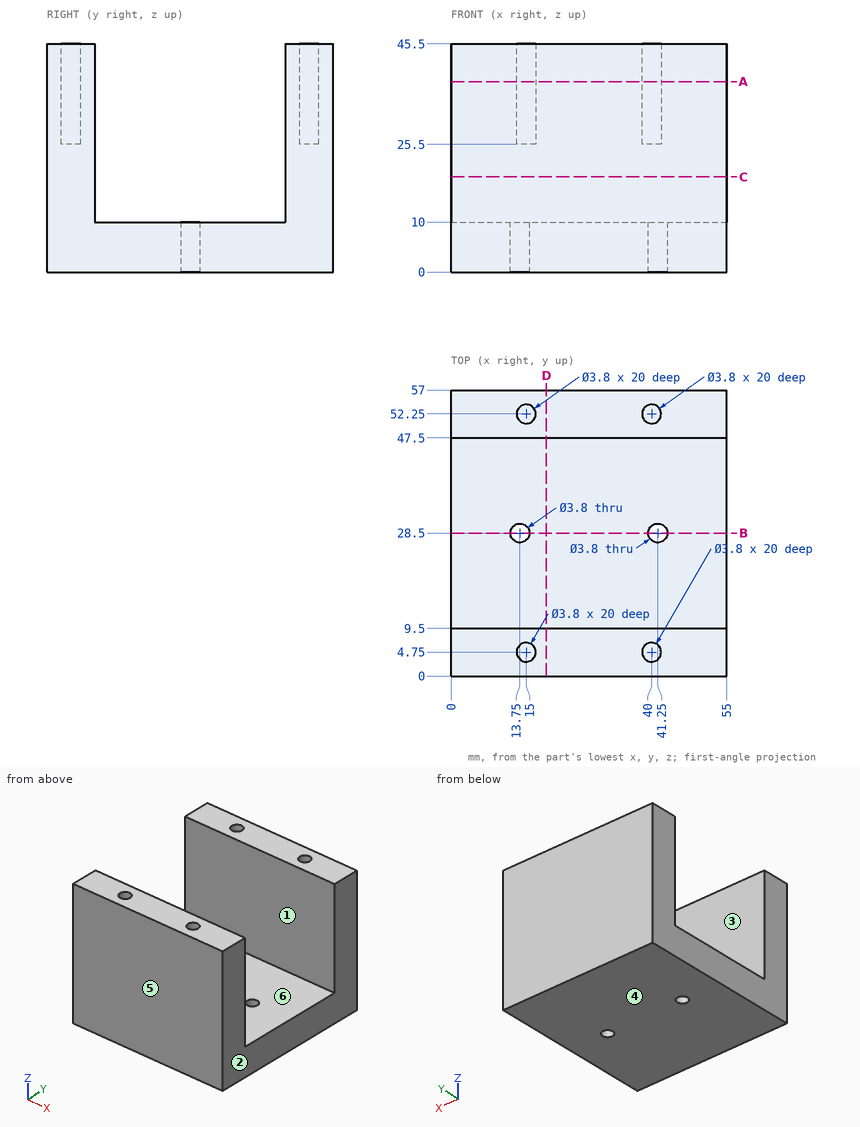
Could you check a few things on this drawing? It's one solid part, dimensions in mm from its lowest x, y, z. A direction names the side the tool comes from. Give positions to 0.01 mm unless a question says otherwise; leave off trailing zeros. Order: outer loops, then holes, each group sorted by start corner. A loop starts at its lowest first (then second) coordinate and runs counter-clockwise, first axis right, second up. Notation, with made-up numbers: (53, -21) - (81, -21) arc R25 ccw to (81, -2) - close; hole circle Ø8 at (47.25, -0.5). An arc over 180 degrees is marked (long way). Return JSON: item names as keys, results as strings. Group by question number.
Q1. Suppose I cut it at A-A, the plane z = 38. Please give me the cut outline in (x, y), and give its area (4 significant figures).
Q2. Please list where these lines run through material, in increasing order: line 1 along Y through (x, z) = (15, 33.75); line 2 along X through (y, z) = (52, 32.5); line 3 along Y through (x, z) = (20, 34). Write a range as [from, to].
Q3. Suppose I cut it at B-B, the plane y = 28.5. Please give me the cut outline in (x, z), and give its area (3 significant figures).
Q4. Thinking about a two-plate mould opening in Y: for the marked faces 3, 4, 5 and 6, which applies, pulls with the +Y half, pulls with the -Y half, needs draft (parallel to the pull), parting line crosses it, or undercut?
Q5. Which directions (+Z, -Z, +X, -X, +Y, -Y) give clear straight access to the entire face, cutting with the end or side of a thin tool? Please do the marked faces 1 and 2.
Q6. Suppose I cut it at C-C, the plane z = 19. Please give me the cut outline in (x, y), and give its area (4 significant figures).
Q7. Will these pins go through, and if not, where does the flat tip stop? pin 1 Ø1 at (x, y) = (41.5, 41.5) entering from +Z; pin 2 Ø6 at (x, y) = (28.5, 12) entering from +Z; pin 3 Ø3.5 at (x, y) = (15, 4.75) entering from +Z; pin 4 Ø3 at (y, z) = (34.5, 13) entering from +X.
Q8. Suppose I cut it at D-D, the plane x = 19. Please give me the cut outline in (y, z).
Resolved:
{
 "1": {"outline": "(0, 0) - (55, 0) - (55, 9.5) - (0, 9.5) - close; (0, 47.5) - (55, 47.5) - (55, 57) - (0, 57) - close; hole circle Ø3.8 at (15, 4.75); hole circle Ø3.8 at (15, 52.25); hole circle Ø3.8 at (40, 4.75); hole circle Ø3.8 at (40, 52.25)", "area": "1,000 mm2"},
 "2": {"line 1": "y = [0, 2.85], [6.65, 9.5], [47.5, 50.35], [54.15, 57]", "line 2": "x = [0, 13.12], [16.88, 38.12], [41.88, 55]", "line 3": "y = [0, 9.5], [47.5, 57]"},
 "3": {"outline": "(0, 0) - (11.85, 0) - (11.85, 10) - (0, 10) - close; (15.65, 0) - (39.35, 0) - (39.35, 10) - (15.65, 10) - close; (43.15, 0) - (55, 0) - (55, 10) - (43.15, 10) - close", "area": "474 mm2"},
 "4": {"face 3": "undercut", "face 4": "needs draft", "face 5": "pulls with the -Y half", "face 6": "undercut"},
 "5": {"face 1": "+Z, +X, -X", "face 2": "+Z, -Z, +X, +Y, -Y"},
 "6": {"outline": "(0, 0) - (55, 0) - (55, 9.5) - (0, 9.5) - close; (0, 47.5) - (55, 47.5) - (55, 57) - (0, 57) - close", "area": "1,045 mm2"},
 "7": {"pin 1": "stops at z = 10", "pin 2": "stops at z = 45.5", "pin 3": "stops at z = 25.5", "pin 4": "passes through"},
 "8": {"outline": "(0, 0) - (57, 0) - (57, 45.5) - (47.5, 45.5) - (47.5, 10) - (9.5, 10) - (9.5, 45.5) - (0, 45.5) - close"}
}
